Design review of the part built by this model. Coordinates are the model's own, in mm. A direction names the side the tool comes from. Give positions to 0.01 mm unless a question says otherwise; leave off trailing zeros. Write each loop counter-clockwise with the first axis right and the second up, starting at its lowest first coordinate (ties: lowest second). Pieces come first, ordered by that corner, then holes. Notation, with made-up numbers: (48.25, -2) -> (61.25, -2) arc R12 ccw to (61.25, 20) -> close; hole circle Ø6 at (46, 51.25). An arc over 180 degrees is marked (long way). Put each result on its own line as item: value. Start each with the question number.
Autodesk Inventor part; units mm, degrees
ref_plane "YZ Plane" through (0, 0, 0) normal (1, 0, 0) x (0, 1, 0)
ref_plane "XZ Plane" through (0, 0, 0) normal (0, 1, 0) x (-1, 0, 0)
ref_plane "XY Plane" through (0, 0, 0) normal (0, 0, 1) x (1, 0, 0)
sketch "Sketch1" plane through (0, 0, 0) normal (0, 1, 0) x (-1, 0, 0)
  line L0 (0, 0) -> (150, 0)
  line L1 (150, 0) -> (150, -150)
  line L2 (150, -150) -> (0, -150)
  line L3 (0, -150) -> (0, 0)
  dimension "d0" = 150
  dimension "d1" = 150
extrude "Extrusion1" add sketch "Sketch1" along normal blind 10
sketch "Sketch2" plane through (-150, 0, 0) normal (0, 0, 1) x (1, 0, 0)
  line L0 (0, 0) -> (0, 10)
  line L1 (150, 0) -> (150, 10)
  line L2 (0, 7.5) -> (150, 7.5)
  line L3 (150, 7.5) -> (150, 2.5)
  line L4 (150, 2.5) -> (0, 2.5)
  line L5 (0, 2.5) -> (0, 7.5)
  line L6 (150, 7.5) -> (135, 7.5)
  line L7 (135, 7.5) -> (135, 2.5)
  line L8 (135, 2.5) -> (150, 2.5)
  line L9 (150, 2.5) -> (150, 7.5)
  line L10 (0, 7.5) -> (15, 7.5)
  line L11 (15, 7.5) -> (15, 2.5)
  line L12 (15, 2.5) -> (0, 2.5)
  line L13 (0, 2.5) -> (0, 7.5)
  point P0 (135, 2.5)
  point P1 (135, 7.5)
  dimension "d4" = 5
  dimension "d5" = 15
  dimension "d6" = 5
  dimension "d7" = 15
  dimension "d8" = 5
sketch "Sketch3" plane through (0, 0, 0) normal (1, 0, 0) x (0, 0, -1)
  line L0 (0, 0) -> (0, 10)
  line L1 (0, 7.5) -> (150, 7.5)
  line L2 (150, 7.5) -> (150, 2.5)
  line L3 (150, 2.5) -> (0, 2.5)
  line L4 (0, 2.5) -> (0, 7.5)
  line L5 (0, 7.5) -> (15, 7.5)
  line L6 (15, 7.5) -> (15, 2.5)
  line L7 (15, 2.5) -> (0, 2.5)
  line L8 (0, 2.5) -> (0, 7.5)
  line L9 (150, 7.5) -> (135, 7.5)
  line L10 (135, 7.5) -> (135, 2.5)
  line L11 (135, 2.5) -> (150, 2.5)
  line L12 (150, 2.5) -> (150, 7.5)
  dimension "d9" = 150
  dimension "d10" = 5
  dimension "d11" = 15
  dimension "d12" = 5
  dimension "d13" = 15
  dimension "d14" = 5
extrude "Extrusion2" add sketch "Sketch2" along normal blind 25 contours L11 L2 L7 L4
extrude "Extrusion3" cut sketch "Sketch3" against normal blind 25 contours L6 L1 L10 L3
properties part number "TSU_MF_Floor"
Q1. Take a section at C-C on z = -121.5. Give the boundary of the cut face in (x, y), then the cut area to 4 significant figures.
Q2. For pin 1 (5.5 mm diameter, centred on y = 5, z = -55.5, fed in from +X); pin 2 (4 mm diameter, centred on y = 6, z = 6.5, fed in from +X); pin 3 (5.5 mm diameter, centred on y = 4, z = 6.5, fed in from -X); pin 4 (12.5 mm diameter, centred on x = -103, z = 12, fed in from -Y), all flat-tipped, find the tip position at first contact; note any pin that passes through.
Q3. Machinability: for faces 1 (the face through (-74, 0, -74)), 2 (the face through (-76, 7.5, 12)), 3 (the face through (0, 2, -76)), 4 (the face through (-15, 5, 12)), 5 (the face through (-12, 2.5, -76)), which of the approach directions +Z, -Z, +X, -X, +Y, -Y give a long, thin tool a straight path to every point of the face, cutting with its end or side? Answer none if there is none.
Q4. To check wall thickness, follow probe 1 along X at (y, z) = (7, -73); probe 2 along Z at (x, y) = (-87, 0.5); probe 3 along Y at (x, z) = (-59, 5.5). State the ranges of each line that lie inside material, in increasing order. Write a range as from..to.
Q5. Take a section at B-B on x = -122. Give the boundary of the cut face in (y, z), then the cut area to 4 significant figures.
Q6. Mouldability with a two-part tool opening along Y and no side actions: class faces 6 (the face through (-12, 7.5, -74)), 7 (the face through (-135, 5, 12)), 8 (the face through (-74, 2.5, 12)) as +Y half, -Y half, draft (parallel to the pull), parting line (faces both ways), or undercut.
Q7. Take a section at D-D on y = 4.75. Give the boundary of the cut face in (x, z).
Q8. Take a section at A-A on x = -10.5. Give the boundary of the cut face in (y, z).
Result:
1. outline: (-150, 0) -> (0, 0) -> (0, 2.5) -> (-25, 2.5) -> (-25, 7.5) -> (0, 7.5) -> (0, 10) -> (-150, 10) -> close
1. area: 1,375 mm^2
2. pin 1: stops at x = 0
2. pin 2: stops at x = -15
2. pin 3: stops at x = -135
2. pin 4: stops at y = 2.5
3. face 1: +Z, -Z, +X, -X, -Y
3. face 2: +Z, +X, -X, +Y
3. face 3: +Z, -Z, +X, +Y, -Y
3. face 4: +Z, +X, +Y, -Y
3. face 5: +X
4. probe 1: x = -150..-25
4. probe 2: z = -150..0
4. probe 3: y = 2.5..7.5
5. outline: (0, -150) -> (10, -150) -> (10, 0) -> (7.5, 0) -> (7.5, 25) -> (2.5, 25) -> (2.5, 0) -> (0, 0) -> close
5. area: 1,625 mm^2
6. face 6: undercut
6. face 7: draft
6. face 8: -Y half
7. outline: (-150, -150) -> (0, -150) -> (0, -135) -> (-25, -135) -> (-25, -15) -> (0, -15) -> (0, 0) -> (-15, 0) -> (-15, 25) -> (-135, 25) -> (-135, 0) -> (-150, 0) -> close
8. outline: (0, -150) -> (10, -150) -> (10, 0) -> (0, 0) -> close; hole (2.5, -135) -> (7.5, -135) -> (7.5, -15) -> (2.5, -15) -> close
